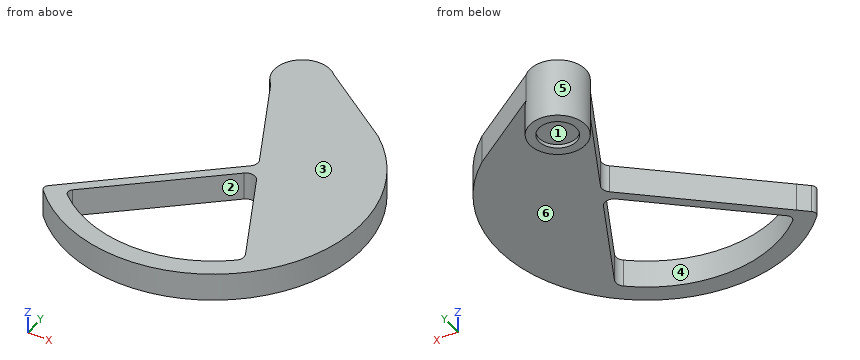
```python
from build123d import *

# Parameters (mm, degrees)
EXTRUDE_1_DEPTH     = 15
EXTRUDE_START       = 17
SKETCH_9_R          = 15
EXTRUDE_3_DEPTH     = 17
SKETCH_10_R         = 10.1
CUT_EXTRUDE_4_DEPTH = 2


with BuildPart() as part:
    # ｽｹｯﾁ4 → ﾎﾞｽ - 押し出し1 (new body)
    with BuildSketch(Plane.XY):
        with BuildLine():
            Line((-53.623111018, -124.995132678), (-58.940636287, -129.45706617))
            ThreePointArc((-58.940636287, -129.45706617), (-60.005384698, -131.552012131), (-59.233530865, -133.771635843))
            ThreePointArc((-59.233530865, -133.771635843), (57.362306223, -135.763481103), (52.076178918, -19.270504783))
            Line((52.076178918, -19.270504783), (10.606601718, 10.606601718))
            ThreePointArc((10.606601718, 10.606601718), (-10.606601718, 10.606601718), (-10.606601718, -10.606601718))
            Line((-10.606601718, -10.606601718), (14.536280154, -62.889638219))
            ThreePointArc((14.536280154, -62.889638219), (14.918089499, -66.109676181), (13.244185189, -68.886809092))
            Line((13.244185189, -68.886809092), (-53.623111018, -124.995132678))
        make_face()
        with BuildLine():
            Line((21.232400696, -76.813798404), (45.844843506, -127.993820346))
            ThreePointArc((45.844843506, -127.993820346), (46.221944165, -131.235480845), (44.518718993, -134.019289696))
            ThreePointArc((44.518718993, -134.019289696), (-2.231208213, -149.964431749), (-47.870174388, -131.072951785))
            ThreePointArc((-47.870174388, -131.072951785), (-48.817477846, -128.802229421), (-47.747678417, -126.586582094))
            Line((-47.747678417, -126.586582094), (13.511229465, -75.151532228))
            ThreePointArc((13.511229465, -75.151532228), (17.77869109, -74.092739753), (21.232400696, -76.813798404))
        make_face(mode=Mode.SUBTRACT)
    extrude(amount=EXTRUDE_1_DEPTH)

    # ｽｹｯﾁ9 → ﾎﾞｽ - 押し出し3 (add)
    with BuildSketch(Plane(origin=(0, 0, 0), x_dir=(-1, 0, 0), z_dir=(0, 0, -1)).offset(EXTRUDE_START)):
        Circle(SKETCH_9_R)
    extrude(amount=-EXTRUDE_3_DEPTH)

    # ｽｹｯﾁ10 → ｶｯﾄ - 押し出し4 (cut)
    with BuildSketch(Plane(origin=(0, 0, -17), x_dir=(-1, 0, 0), z_dir=(0, 0, -1))):
        Circle(SKETCH_10_R)
    extrude(amount=-CUT_EXTRUDE_4_DEPTH, mode=Mode.SUBTRACT)


solid = part.part
```
Geometry check sheet. Reference: the model listing, model coordinates, mm. Face numbers are marked on the shaded views. A direction names the side the tool comes from. Give positions to 0.01 mm unless a question says otherwise; leave off trailing zeros. Order: outer loops, then holes, each group sorted by start corner. A loop starts at its lowest first (then second) coordinate and runs counter-clockwise, first axis right, second up. Notation, with made-up numbers: (-38, -19.75) - (-32, -19.75) arc R20 cw to (-32, 19.25) - close; hole circle Ø9 at (38.5, -32). An arc over 180 degrees is marked (long way). Answer in a Markdown table with one row per item. Add a question column.
Q1. Gauge pin test, flat ends, axial feed: pin 1 (3 mm diameter, centred on x = 10, z = -4, fed in from -Y); pin 2 (1.5 mm diameter, centred on x = -28.5, z = 3.5, fed in from -Y); pin 3 (4 mm diameter, centred on x = -37.5, z = 10, fed in from -Y). Record the tip position at first contact, or that the pin passes through.
Q2. Tool access check on the marked faces 1, 2 and 3. Record the directions out of +Z, -Z, +X, -X, +Y, -Y that give a thin tool (end or side, any length) a straight path to the whole face; none if there is none.
Q3. Mould release check, pull along X, two halves, no side actions. Record for the marked faces 4, 5 and 6: pulls with the +X half, pulls with the -X half, needs draft (parallel to the pull), parting line crosses it, or undercut.
Q4. Cross-section at A-A, the plane y = -110.5. Enter the section's corners in (x, z).
Q5. Cross-section at B-B, the plane z = 11. Enter the section's corners in (x, y), then the cut area to 3 significant figures.
Q6. Cross-section at D-D, the plane x = 24. Enter the section's corners in (y, z), then the cut area to 3 significant figures.
Q7. Cross-section at C-C, the plane x = 0. Enter the section's corners in (y, z).
Q8. Material ranges on probe 1 along Y at (x, z) = (0, -16.4); probe 2 along Z at (x, y) = (-30, -152); probe 3 along X at (y, z) = (-101, 1), recorded low to high. Write a range as from..to.
Check values:
| question | item | result |
|---|---|---|
| 1 | pin 1 | stops at y = -12.36 |
| 1 | pin 2 | stops at y = -155.03 |
| 1 | pin 3 | stops at y = -151.69 |
| 2 | face 1 | -Z |
| 2 | face 2 | +Z, -Z |
| 2 | face 3 | +Z, +X, -X, +Y, -Y |
| 3 | face 4 | undercut |
| 3 | face 5 | parting line crosses it |
| 3 | face 6 | needs draft |
| 4 | outline | (-36.35, 0) - (-28.59, 0) - (-28.59, 15) - (-36.35, 15) - close; (37.43, 0) - (73.96, 0) - (73.96, 15) - (37.43, 15) - close |
| 5 | outline | (-59.23, -133.77) arc R80 ccw (long way) to (52.08, -19.27) - (10.61, 10.61) arc R15 ccw to (-10.61, -10.61) - (14.54, -62.89) arc R5 cw to (13.24, -68.89) - (-58.94, -129.46) arc R3 ccw to start; hole (-47.87, -131.07) arc R70 ccw to (44.52, -134.02) arc R5 ccw to (45.84, -127.99) - (21.23, -76.81) arc R5 ccw to (13.51, -75.15) - (-47.75, -126.59) arc R3 ccw to start |
| 5 | area | 8,940 mm^2 |
| 6 | outline | (-156.32, 0) - (-145.76, 0) - (-145.76, 15) - (-156.32, 15) - close; (-82.57, 0) - (0.96, 0) - (0.96, 15) - (-82.57, 15) - close |
| 6 | area | 1,410 mm^2 |
| 7 | outline | (-160, 0) - (-150, 0) - (-150, 15) - (-160, 15) - close; (-86.5, 0) - (-80, 0) - (-80, 15) - (-86.5, 15) - close; (-32.66, 0) - (-15, 0) - (-15, -17) - (-10.1, -17) - (-10.1, -15) - (10.1, -15) - (10.1, -17) - (15, -17) - (15, 15) - (-32.66, 15) - close |
| 8 | probe 1 | y = -15..-10.1, 10.1..15 |
| 8 | probe 2 | z = 0..15 |
| 8 | probe 3 | x = -25.03..-17.27, 32.86..77.19 |
